from build123d import *

# Parameters (mm, degrees)
SKETCH2_W           = 130
SKETCH2_H           = 60
SKETCH2_W_2         = 5
SKETCH2_H_2         = 3
BOSS_EXTRUDE1_DEPTH = 3


with BuildPart() as part:
    # Sketch2 → Boss-Extrude1 (new body)
    with BuildSketch(Plane.XY):
        Rectangle(SKETCH2_W, SKETCH2_H)
        with Locations((67.5, 28.5)):
            Rectangle(SKETCH2_W_2, SKETCH2_H_2)
        with Locations((-67.5, 28.5)):
            Rectangle(SKETCH2_W_2, SKETCH2_H_2)
    extrude(amount=BOSS_EXTRUDE1_DEPTH)


solid = part.part
The model under review builds one solid part; all positions refer to its coordinate system, in mm. A direction names the side the tool comes from. Give positions to 0.01 mm unless a question says otherwise; leave off trailing zeros. Write each loop counter-clockwise with the first axis right and the second up, starting at its lowest first coordinate (ties: lowest second). Pieces come first, ordered by that corner, then holes. Notation, with made-up numbers: M 34,45 L 87,45 A28 ccw 87,81 Z; hole C 24.5,30 d8. An arc over 180 degrees is marked long. One line per question, with ' | ' between items. Start each with the question number.
Item 1: Wall thickness on line 1 (X direction, y = -18, z = 0.6): over which ranges is the line inside the solid? List them lowest first. Write a range as from..to.
Item 2: For faces 1 (the flat face through (67, 27, 1)), 2 (the flat face through (-68, 27, 1)), 3 (the flat face through (-70, 28, 1)), list the 3-axis set-ups (+Z, -Z, +X, -X, +Y, -Y) from which the entire face can be reached by the end or side of a thin tool; tool diameter is ignored.
Item 3: We need section A-A on z = 1.1. Write out the cut boundary in (x, y), plus the area to 3 significant figures.
Item 4: We need section B-B on y = 14. Write out the cut boundary in (x, z), plus the area to 3 significant figures.
Item 5: For pin 1 (1 mm diameter, centred on y = -4.5, z = 1.5, fed in from +X); pin 2 (1.5 mm diameter, centred on x = -67.5, z = 1.5, fed in from -Y); pin 3 (1.5 mm diameter, centred on y = -11, z = 1, fed in from -X), all flat-tipped, find the tip position at first contact; note any pin that passes through.
Results found:
1) line 1: x = -65..65
2) face 1: +Z, -Z, +X, -Y | face 2: +Z, -Z, -X, -Y | face 3: +Z, -Z, -X, +Y, -Y
3) outline: M -70,27 L -65,27 L -65,-30 L 65,-30 L 65,27 L 70,27 L 70,30 L -70,30 Z | area: 7,830 mm2
4) outline: M -65,0 L 65,0 L 65,3 L -65,3 Z | area: 390 mm2
5) pin 1: stops at x = 65 | pin 2: stops at y = 27 | pin 3: stops at x = -65
